from build123d import *

# Parameters (mm, degrees)
F0_W     = 90
F0_H     = 15
F1_DEPTH = 5
F2_W     = 90
F2_H     = 13
F3_DEPTH = 15
F5_D     = 4.2
F5_DEPTH = 8
F5_TIP   = 1.2618073
F7_D     = 4.2
F7_DEPTH = 8
F7_TIP   = 1.2618073
F8_SIZE  = 1


with BuildPart() as f1:
    # F0 (on Top) → F1 (new body)
    with BuildSketch(Plane.XY):
        with Locations((45, 7.5)):
            Rectangle(F0_W, F0_H)
    extrude(amount=F1_DEPTH)

    # F2 (on face) → F3 (join)
    with BuildSketch(Plane.XY.offset(5)):
        with Locations((45, 8.5)):
            Rectangle(F2_W, F2_H)
    extrude(amount=F3_DEPTH)

    # F5
    with Locations(Plane.YZ.offset(90)):
        with Locations((7.5, 10)):
            Hole(F5_D / 2, depth=F5_DEPTH)
            with Locations((0, 0, -(F5_DEPTH + F5_TIP / 2))):  # 118° drill point
                Cone(0, F5_D / 2, F5_TIP, mode=Mode.SUBTRACT)

    # F7
    with Locations(Plane(origin=(0, 0, 0), x_dir=(0, -1, 0), z_dir=(-1, 0, 0))):
        with Locations((-7.5, 10)):
            Hole(F7_D / 2, depth=F7_DEPTH)
            with Locations((0, 0, -(F7_DEPTH + F7_TIP / 2))):  # 118° drill point
                Cone(0, F7_D / 2, F7_TIP, mode=Mode.SUBTRACT)

    # F8
    f8_edges = [f1.edges().sort_by_distance(p)[0] for p in [
        (45, 2, 20),
        (90, 8.5, 20),
        (45, 15, 20),
        (0, 8.5, 20),
    ]]
    chamfer(f8_edges, length=F8_SIZE)


solid = f1.part
Work out the finished part from the listing and answer in its coordinate system (mm). A direction names the side the tool comes from. Give positions to 0.01 mm unless a question says otherwise; leave off trailing zeros. Loops run counter-clockwise (first coordinate to the right, second up) from the corner with the lowest first, then second, coordinate; pieces in that order, holes last. Notation, with made-up numbers: (8.25, -5) - (22.25, -5) arc R22 cw to (22.25, 16) - close; hole circle Ø1 at (52, 19). An arc over 180 degrees is marked (long way). Answer in a Markdown table with one row per item.
(1) Flat-ended cylindrical pins translate along their axes: pin 1 Ø0.6 at (x, y) = (32, 1) entering from +Z; pin 2 Ø3.5 at (y, z) = (7.5, 10) entering from +X; pin 3 Ø3 at (y, z) = (6, 14) entering from -X; pin 4 Ø4 at (x, z) = (46.5, 10.5) entering from -Y. Find the tip coordinate at first contact, or state that the pin passes through.
Results list:
| item | result |
|---|---|
| pin 1 | stops at z = 5 |
| pin 2 | stops at x = 81.79 |
| pin 3 | stops at x = 0 |
| pin 4 | stops at y = 2 |
(2) Consider L1, parallel to Y at x = 86, z = 10; L2, parallel to Z at x = 6, y = 7.5; L3, parallel to Y at x = 28.5, z = 8. Determine where each line is inside the solid, lowest interval first. Write a range as [from, to].
Results list:
| item | result |
|---|---|
| L1 | y = [2, 5.4], [9.6, 15] |
| L2 | z = [0, 7.9], [12.1, 20] |
| L3 | y = [2, 15] |
(3) Section A-A (x = 20) is taken. Give the vertices of the cut face in (y, z).
Results list:
| item | result |
|---|---|
| outline | (0, 0) - (15, 0) - (15, 19) - (14, 20) - (3, 20) - (2, 19) - (2, 5) - (0, 5) - close |
(4) A tool of negligible diameter and unlimited length cuts with its end or side. For faces 5 (the face through (44, 2, 12)), 6 (the face through (9.043, 7.547, 10.362)), from which of +Z, -Z, +X, -X, +Y, -Y can it reach the whole face along a straight path? Write none if from no direction.
Results list:
| item | result |
|---|---|
| face 5 | +Z, +X, -X, -Y |
| face 6 | -X |
(5) For a pull along Y with two mould halves and no side action, classify faces 1 (the face through (44, 0, 2)), 2 (the face through (44, 9, 20)), 3 (the face through (4.056, 7.227, 12.082)), 4 (the face through (85.944, 7.773, 12.082)) as pulls with the +Y half, pulls with the -Y half, needs draft (parallel to the pull), parting line crosses it, or undercut.
Results list:
| item | result |
|---|---|
| face 1 | pulls with the -Y half |
| face 2 | needs draft |
| face 3 | undercut |
| face 4 | undercut |
(6) Section C-C (z = 16) is taken. Give the vertices of the cut face in (x, y).
Results list:
| item | result |
|---|---|
| outline | (0, 2) - (90, 2) - (90, 15) - (0, 15) - close |
(7) Section B-B (y = 1) is taken. Give the vertices of the cut face in (x, z), and give its area (3 significant figures).
Results list:
| item | result |
|---|---|
| outline | (0, 0) - (90, 0) - (90, 5) - (0, 5) - close |
| area | 450 mm² |
